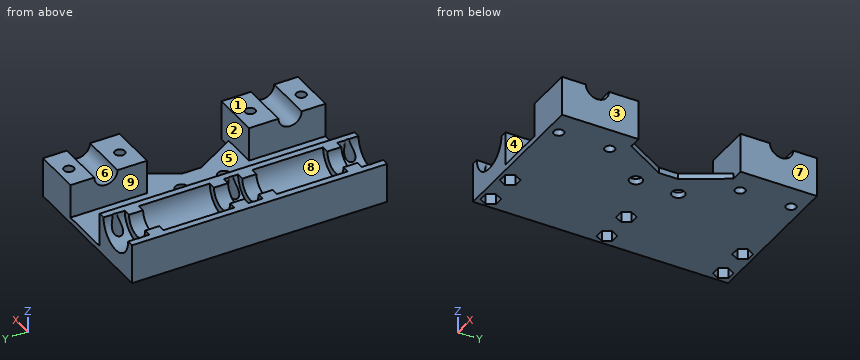
```python
from build123d import *

# Parameters (mm, degrees)
PAD003_DEPTH    = 5
PAD001_DEPTH    = 5
PAD002_DEPTH    = 5
PAD004_DEPTH    = 5
SKETCH_W        = 55
SKETCH_H        = 90
PAD_DEPTH       = 14
SKETCH001_R     = 7.6
POCKET_DEPTH    = 90.001
SKETCH002_R     = 1.75
POCKET001_DEPTH = 14.001
POCKET002_DEPTH = 12
SKETCH004_R     = 2.25
POCKET003_DEPTH = 14.001
SKETCH008_R     = 4.1
POCKET005_DEPTH = 20
POCKET007_DEPTH = 4.5
POCKET008_DEPTH = 12.5


with BuildPart() as pad003:
    # Sketch020 → Pad003 (new body)
    with BuildSketch(Plane.XZ.offset(-32.5)):
        with BuildLine():
            ThreePointArc((-7.6, 14), (0, 6.4), (7.6, 14))
            Line((7.6, 14), (5, 14))
            ThreePointArc((-5, 14), (0, 9), (5, 14))
            Line((-7.6, 14), (-5, 14))
        make_face()
    extrude(amount=-PAD003_DEPTH)


with BuildPart() as pad001:
    # Sketch018 → Pad001 (new body)
    with BuildSketch(Plane.XZ.offset(-7.5)):
        with BuildLine():
            ThreePointArc((-7.6, 14), (0, 6.4), (7.6, 14))
            Line((7.6, 14), (5, 14))
            ThreePointArc((-5, 14), (0, 9), (5, 14))
            Line((-7.6, 14), (-5, 14))
        make_face()
    extrude(amount=PAD001_DEPTH)


with BuildPart() as pad002:
    # Sketch019 → Pad002 (new body)
    with BuildSketch(Plane.XZ.offset(7.5)):
        with BuildLine():
            ThreePointArc((-7.6, 14), (0, 6.4), (7.6, 14))
            Line((7.6, 14), (5, 14))
            ThreePointArc((-5, 14), (0, 9), (5, 14))
            Line((-7.6, 14), (-5, 14))
        make_face()
    extrude(amount=-PAD002_DEPTH)


with BuildPart() as pad004:
    # Sketch021 → Pad004 (new body)
    with BuildSketch(Plane.XZ.offset(32.5)):
        with BuildLine():
            ThreePointArc((-7.6, 14), (0, 6.4), (7.6, 14))
            Line((7.6, 14), (5, 14))
            ThreePointArc((-5, 14), (0, 9), (5, 14))
            Line((-7.6, 14), (-5, 14))
        make_face()
    extrude(amount=PAD004_DEPTH)


with BuildPart() as fusion:
    # Sketch → Pad (new body)
    with BuildSketch(Plane.XY):
        with Locations((17.5, 0)):
            Rectangle(SKETCH_W, SKETCH_H)
    extrude(amount=PAD_DEPTH)

    # Sketch001 → Pocket (cut, through all)
    with BuildSketch(Plane.XZ.offset(45)):
        with Locations((0, 14)):
            Circle(SKETCH001_R)
    extrude(amount=-POCKET_DEPTH, mode=Mode.SUBTRACT)

    # Sketch002 → Pocket001 (cut, through all)
    with BuildSketch(Plane.XY.offset(14)):
        with Locations((-6, 41)):
            Circle(SKETCH002_R)
        with Locations((-6, -41)):
            Circle(SKETCH002_R)
        with Locations((6, 41)):
            Circle(SKETCH002_R)
        with Locations((6, -41)):
            Circle(SKETCH002_R)
        with Locations((6, 0)):
            Circle(SKETCH002_R)
        with Locations((-6, 0)):
            Circle(SKETCH002_R)
        with Locations((36, 41)):
            Circle(SKETCH002_R)
        with Locations((36, 23)):
            Circle(SKETCH002_R)
        with Locations((36, -23)):
            Circle(SKETCH002_R)
        with Locations((36, -41)):
            Circle(SKETCH002_R)
    extrude(amount=-POCKET001_DEPTH, mode=Mode.SUBTRACT)

    # Sketch003 → Pocket002 (cut)
    with BuildSketch(Plane.XY.offset(14)):
        Polygon((10, 50), (10, -50), (28, -50), (28, -18), (48, -18), (48, 18), (28, 18), (28, 50), align=None)
    extrude(amount=-POCKET002_DEPTH, mode=Mode.SUBTRACT)

    # Sketch004 → Pocket003 (cut, through all)
    with BuildSketch(Plane(origin=(0, 0, 0), x_dir=(1, 0, 0), z_dir=(0, 0, -1))):
        with Locations((25, 7.5)):
            Circle(SKETCH004_R)
        with Locations((25, -7.5)):
            Circle(SKETCH004_R)
    extrude(amount=-POCKET003_DEPTH, mode=Mode.SUBTRACT)

    # Sketch008 → Pocket005 (cut)
    with BuildSketch(Plane.YZ.offset(45)):
        with Locations((-32.5, 14)):
            Circle(SKETCH008_R)
        with Locations((32.5, 14)):
            Circle(SKETCH008_R)
    extrude(amount=-POCKET005_DEPTH, mode=Mode.SUBTRACT)

    # Sketch012 → Pocket007 (cut)
    with BuildSketch(Plane(origin=(0, 0, 0), x_dir=(1, 0, 0), z_dir=(0, 0, -1))):
        Polygon((-4.412285, 2.750003), (-7.587715, 2.750003), (-9.17543, 0), (-7.587715, -2.750003), (-4.412285, -2.750003), (-2.82457, 0), align=None)
        Polygon((7.587715, 2.750003), (4.412285, 2.750003), (2.82457, 0), (4.412285, -2.750003), (7.587715, -2.750003), (9.17543, 0), align=None)
        Polygon((-4.412285, 43.750003), (-7.587715, 43.750003), (-9.17543, 41), (-7.587715, 38.249997), (-4.412285, 38.249997), (-2.82457, 41), align=None)
        Polygon((7.587715, -38.249997), (4.412285, -38.249997), (2.82457, -41), (4.412285, -43.750003), (7.587715, -43.750003), (9.17543, -41), align=None)
        Polygon((7.587715, 43.750003), (4.412285, 43.750003), (2.82457, 41), (4.412285, 38.249997), (7.587715, 38.249997), (9.17543, 41), align=None)
        Polygon((-4.412285, -38.249997), (-7.587715, -38.249997), (-9.17543, -41), (-7.587715, -43.750003), (-4.412285, -43.750003), (-2.82457, -41), align=None)
    extrude(amount=-POCKET007_DEPTH, mode=Mode.SUBTRACT)

    # Sketch022 → Pocket008 (cut, symmetric)
    with BuildSketch(Plane.XY.offset(2)):
        Polygon((40.573685, 18), (32, 3.425), (32, -3.425), (40.573685, -18), (51.573685, -18), (51.573685, 18), align=None)
    extrude(amount=POCKET008_DEPTH, both=True, mode=Mode.SUBTRACT)

    # Fusion: union Pad003, Pad001, Pad002, Pad004
    add(pad003.part)
    add(pad001.part)
    add(pad002.part)
    add(pad004.part)


solid = fusion.part
```
Source: CAD feature listing. Evaluate the final solid. Frame: model axes, mm. Face numbers are marked on the shaded views. A direction names the side the tool comes from. Round coordinates to 2 decimals unless told otherwise and drop trailing zeros. Loops run counter-clockwise (first coordinate to the right, second up) from the corner with the lowest first, then second, coordinate; pieces in that order, holes last. Notation, with made-up numbers: M 21.5,4.5 L 26.5,4.5 A14 cw 26.5,17.5 Z; hole C 56,12.25 d9. An arc over 180 degrees is marked long. Use a Markdown table: item, result. Add a question column.
1. Ray query, line 1 along Y through (x, z) = (6, 10.75); line 2 along Y through (x, z) = (36, 8.75); line 3 along Y through (x, z) = (25, 0.55). Return the intervals inside material, ascending. Write a range as [from, to].
2. Cut plane B-B, the plane x = 25. Output: boundary loops of the cut face in (y, z).
3. Pull-direction query (X, two-part tool) for the marked faces 6, 7, 8 and 9; classes: +X half, -X half, draft (parallel to the pull), parting line (faces both ways), or undercut.
4. Cut plane A-A, the plane y = -23. Output: boundary loops of the cut face in (x, z), and give its area (3 significant figures).
5. Cut plane D-D, the plane z = 12.5. State how many separate pieces and enclosed holes the cut face has, and give its area (3 significant figures).
6. Contact query for flat-ended pins moving along their axis: pin 1 (4 mm diameter, centred on y = 1, z = 1.5, fed in from +X); pin 2 (4 mm diameter, centred on x = -6, y = 0, fed in from -Z); pin 3 (5 mm diameter, centred on x = 34, y = -10.5, fed in from +Z). Output: stop coordinate, or through.
7. Set-up query: the marked faces 1, 2, 3, 4 and 5. Return all of +Z, -Z, +X, -X, +Y, -Y with unobstructed straight access to the full face (end or side cutting, diameter ignored); none if empty.
8. Cut plane C-C, the plane x = 0. Output: boundary loops of the cut face in (y, z), and give its area (3 significant figures).
Solution:
| question | item | result |
|---|---|---|
| 1 | line 1 | y = [-37.5, -32.5], [-7.5, -2.5], [2.5, 7.5], [32.5, 37.5] |
| 1 | line 2 | y = [-45, -42.75], [-39.25, -24.75], [-21.25, -18], [18, 21.25], [24.75, 39.25], [42.75, 45] |
| 1 | line 3 | y = [-45, -9.75], [-5.25, 5.25], [9.75, 45] |
| 2 | outline | M -45,0 L -9.75,0 L -9.75,2 L -45,2 Z; M -5.25,0 L 5.25,0 L 5.25,2 L -5.25,2 Z; M 9.75,0 L 45,0 L 45,2 L 9.75,2 Z |
| 3 | face 6 | draft |
| 3 | face 7 | +X half |
| 3 | face 8 | undercut |
| 3 | face 9 | undercut |
| 4 | outline | M -10,0 L 34.25,0 L 34.25,14 L 28,14 L 28,2 L 10,2 L 10,14 L 7.6,14 A7.6 cw -7.6,14 L -10,14 Z; M 37.75,0 L 45,0 L 45,14 L 37.75,14 Z |
| 4 | area | 414 mm2 |
| 5 | separate pieces | 6 |
| 5 | enclosed holes | 4 |
| 5 | area | 1,180 mm2 |
| 6 | pin 1 | stops at x = 32 |
| 6 | pin 2 | stops at z = 4.5 |
| 6 | pin 3 | stops at z = 2 |
| 7 | face 1 | +Z, +X, -X, +Y, -Y |
| 7 | face 2 | +Z, +X |
| 7 | face 3 | +Z, -Z, +X, +Y, -Y |
| 7 | face 4 | +Z, +Y, -Y |
| 7 | face 5 | +Z |
| 8 | outline | M -45,0 L 45,0 L 45,6.4 L 37.5,6.4 L 37.5,9 L 32.5,9 L 32.5,6.4 L 7.5,6.4 L 7.5,9 L 2.5,9 L 2.5,6.4 L -2.5,6.4 L -2.5,9 L -7.5,9 L -7.5,6.4 L -32.5,6.4 L -32.5,9 L -37.5,9 L -37.5,6.4 L -45,6.4 Z |
| 8 | area | 628 mm2 |
